from build123d import *

# Parameters (mm, degrees)
BOX024_W                = 6
BOX024_H                = 36
BOX024_DEPTH            = 23
CYLINDER011_R           = 2.75
CYLINDER011_DEPTH       = 74.5
CYLINDER011_PITCH_ANGLE = 90
CYLINDER008_R           = 1.75
CYLINDER008_DEPTH       = 21.5
CYLINDER008_PITCH_ANGLE = 90
CYLINDER009_R           = 3
CYLINDER009_DEPTH       = 21.5
CYLINDER009_PITCH_ANGLE = 90
BOX007_W                = 3
BOX007_H                = 56
BOX007_DEPTH            = 6
BOX008_W                = 3
BOX008_H                = 56
BOX008_DEPTH            = 6
BOX006_W                = 4
BOX006_H                = 56
BOX006_DEPTH            = 21
CYLINDER003_R           = 1.75
CYLINDER003_DEPTH       = 74.5
CYLINDER003_PITCH_ANGLE = 90
BOX003_W                = 28
BOX003_H                = 88
BOX003_DEPTH            = 38
BOX002_W                = 28
BOX002_H                = 88
BOX002_DEPTH            = 38
BOX001_W                = 47
BOX001_H                = 42
BOX001_DEPTH            = 25
BOX_W                   = 72
BOX_H                   = 58
BOX_DEPTH               = 24
FILLET_R                = 10
CHAMFER_SIZE            = 3


with BuildPart() as cube024:
    # Box024 → Box024 (new body)
    with BuildSketch(Plane(origin=(0, 19, 7), x_dir=(1, 0, 0), z_dir=(0, 0, 1))):
        with Locations((3, 18)):
            Rectangle(BOX024_W, BOX024_H)
    extrude(amount=BOX024_DEPTH)


with BuildPart() as joint_d013:
    # Cylinder011 → Cylinder011 (new body)
    with BuildSketch(Plane.XY):
        Circle(CYLINDER011_R)
    extrude(amount=CYLINDER011_DEPTH)


with BuildPart() as joint_d013_1:
    # Cylinder011 pitch: moved
    add(joint_d013.part.rotate(Axis((0, 0, 0), (0, 1, 0)), CYLINDER011_PITCH_ANGLE))


with BuildPart() as joint_d013_2:
    # Cylinder011 placement: moved
    add(joint_d013_1.part.moved(Location((-3, 9.5, 12))))


with BuildPart() as joint_d010:
    # Cylinder008 → Cylinder008 (new body)
    with BuildSketch(Plane.XY):
        Circle(CYLINDER008_R)
    extrude(amount=CYLINDER008_DEPTH)


with BuildPart() as joint_d010_1:
    # Cylinder008 pitch: moved
    add(joint_d010.part.rotate(Axis((0, 0, 0), (0, 1, 0)), CYLINDER008_PITCH_ANGLE))


with BuildPart() as joint_d010_2:
    # Cylinder008 placement: moved
    add(joint_d010_1.part.moved(Location((16, -24.5, 7))))


with BuildPart() as joint_d011:
    # Cylinder009 → Cylinder009 (new body)
    with BuildSketch(Plane.XY):
        Circle(CYLINDER009_R)
    extrude(amount=CYLINDER009_DEPTH)


with BuildPart() as joint_d011_1:
    # Cylinder009 pitch: moved
    add(joint_d011.part.rotate(Axis((0, 0, 0), (0, 1, 0)), CYLINDER009_PITCH_ANGLE))


with BuildPart() as joint_d011_2:
    # Cylinder009 placement: moved
    add(joint_d011_1.part.moved(Location((32, -24.5, 7))))


with BuildPart() as fusion001:
    # Fusion001 base: copy of Joint-D011
    add(joint_d011_2.part)

    # Fusion001: union Joint-D010
    add(joint_d010_2.part)


with BuildPart() as fusion002:
    # Fusion002 base: copy of Joint-D011
    add(joint_d011_2.part)

    # Fusion002: union Joint-D010
    add(joint_d010_2.part)


with BuildPart() as fusion002_1:
    # Fusion002 placement: moved
    add(fusion002.part.moved(Location((0, 0, 10))))


with BuildPart() as fusion003:
    # Fusion003 base: copy of Joint-D011
    add(joint_d011_2.part)

    # Fusion003: union Joint-D010
    add(joint_d010_2.part)


with BuildPart() as fusion003_1:
    # Fusion003 placement: moved
    add(fusion003.part.moved(Location((0, 49, 0))))


with BuildPart() as fusion004:
    # Fusion004 base: copy of Joint-D011
    add(joint_d011_2.part)

    # Fusion004: union Joint-D010
    add(joint_d010_2.part)


with BuildPart() as fusion004_1:
    # Fusion004 placement: moved
    add(fusion004.part.moved(Location((0, 49, 10))))


with BuildPart() as cube007:
    # Box007 → Box007 (new body)
    with BuildSketch(Plane(origin=(18.5, -28, 4), x_dir=(1, 0, 0), z_dir=(0, 0, 1))):
        with Locations((1.5, 28)):
            Rectangle(BOX007_W, BOX007_H)
    extrude(amount=BOX007_DEPTH)


with BuildPart() as cube008:
    # Box008 → Box008 (new body)
    with BuildSketch(Plane(origin=(18.5, -28, 14), x_dir=(1, 0, 0), z_dir=(0, 0, 1))):
        with Locations((1.5, 28)):
            Rectangle(BOX008_W, BOX008_H)
    extrude(amount=BOX008_DEPTH)


with BuildPart() as cube006:
    # Box006 → Box006 (new body)
    with BuildSketch(Plane(origin=(25.5, -28, 2), x_dir=(1, 0, 0), z_dir=(0, 0, 1))):
        with Locations((2, 28)):
            Rectangle(BOX006_W, BOX006_H)
    extrude(amount=BOX006_DEPTH)


with BuildPart() as joint_d005:
    # Cylinder003 → Cylinder003 (new body)
    with BuildSketch(Plane.XY):
        Circle(CYLINDER003_R)
    extrude(amount=CYLINDER003_DEPTH)


with BuildPart() as joint_d005_1:
    # Cylinder003 pitch: moved
    add(joint_d005.part.rotate(Axis((0, 0, 0), (0, 1, 0)), CYLINDER003_PITCH_ANGLE))


with BuildPart() as joint_d005_2:
    # Cylinder003 placement: moved
    add(joint_d005_1.part.moved(Location((-22, 9.5, 12))))


with BuildPart() as cube003:
    # Box003 → Box003 (new body)
    with BuildSketch(Plane(origin=(-33, -45, 1), x_dir=(1, 0, 0), z_dir=(0, 0, 1))):
        with Locations((14, 44)):
            Rectangle(BOX003_W, BOX003_H)
    extrude(amount=BOX003_DEPTH)


with BuildPart() as cube002:
    # Box002 → Box002 (new body)
    with BuildSketch(Plane(origin=(37, -45, 1), x_dir=(1, 0, 0), z_dir=(0, 0, 1))):
        with Locations((14, 44)):
            Rectangle(BOX002_W, BOX002_H)
    extrude(amount=BOX002_DEPTH)


with BuildPart() as cube001:
    # Box001 → Box001 (new body)
    with BuildSketch(Plane(origin=(-1, -21, 2), x_dir=(1, 0, 0), z_dir=(0, 0, 1))):
        with Locations((23.5, 21)):
            Rectangle(BOX001_W, BOX001_H)
    extrude(amount=BOX001_DEPTH)


with BuildPart() as pie_d:
    # Box → Box (new body)
    with BuildSketch(Plane(origin=(-15, -29, -3), x_dir=(1, 0, 0), z_dir=(0, 0, 1))):
        with Locations((36, 29)):
            Rectangle(BOX_W, BOX_H)
    extrude(amount=BOX_DEPTH)

    # Cut: cut Cube001
    add(cube001.part, mode=Mode.SUBTRACT)

    # Cut001: cut Cube002
    add(cube002.part, mode=Mode.SUBTRACT)

    # Cut002: cut Cube003
    add(cube003.part, mode=Mode.SUBTRACT)

    # Fillet
    fillet_edges = [pie_d.edges().sort_by_distance(p)[0] for p in [
        (-15, -29, -1),
        (-15, 29, -1),
        (57, -29, -1),
        (57, 29, -1),
    ]]
    fillet(fillet_edges, radius=FILLET_R)

    # Chamfer
    chamfer_edges = [pie_d.edges().sort_by_distance(p)[0] for p in [
        (-5, 0, 21),
        (37, 25, 21),
        (37, -25, 21),
    ]]
    chamfer(chamfer_edges, length=CHAMFER_SIZE)

    # Cut008: cut Joint-D005
    add(joint_d005_2.part, mode=Mode.SUBTRACT)

    # Cut010: cut Cube006
    add(cube006.part, mode=Mode.SUBTRACT)

    # Cut011: cut Cube008
    add(cube008.part, mode=Mode.SUBTRACT)

    # Cut012: cut Cube007
    add(cube007.part, mode=Mode.SUBTRACT)

    # Cut013: cut Fusion004
    add(fusion004_1.part, mode=Mode.SUBTRACT)

    # Cut014: cut Fusion003
    add(fusion003_1.part, mode=Mode.SUBTRACT)

    # Cut015: cut Fusion002
    add(fusion002_1.part, mode=Mode.SUBTRACT)

    # Cut016: cut Fusion001
    add(fusion001.part, mode=Mode.SUBTRACT)

    # Cut017: cut Joint-D013
    add(joint_d013_2.part, mode=Mode.SUBTRACT)

    # Cut039: cut Cube024
    add(cube024.part, mode=Mode.SUBTRACT)


with BuildPart() as pie_d_1:
    # Cut039 placement: moved
    add(pie_d.part.moved(Location((0, 0, 1))))


with BuildPart() as pie_i:
    # Part__Mirroring006: instance of pie-D
    add(pie_d_1.part.mirror(Plane(origin=(0, 0, 0), x_dir=(1, 0, 0), z_dir=(0, 1, 0))))


with BuildPart() as pie_i_1:
    # Part__Mirroring006 placement: moved
    add(pie_i.part.moved(Location((0, 72, 0))))


solid = pie_i_1.part
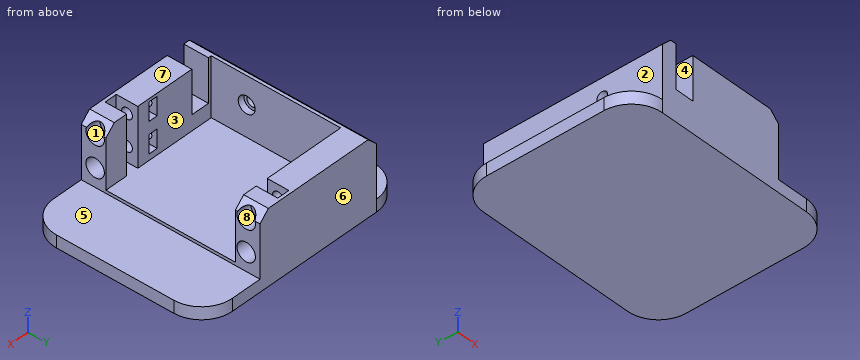
Here's how the part is built. I have some questions about the finished solid (model axes, mm). Face numbers are marked on the shaded views. A direction names the side the tool comes from. Round coordinates to 2 decimals unless told otherwise and drop trailing zeros. Write each loop counter-clockwise with the first axis right and the second up, starting at its lowest first coordinate (ties: lowest second). Pieces come first, ordered by that corner, then holes. Notation, with made-up numbers: (-21.5, 66) -> (31.5, 66) arc R7 cw to (31.5, 72) -> close; hole circle Ø6 at (-31, 80.25). An arc over 180 degrees is marked (long way). One line per item, written item: value.
1) Suppose I cut it at A-A on z = 13. List the corners of the cut face in (x, y) for me.
Filled sheet:
outline: (-5, 43) -> (0, 43) -> (0, 51) -> (-1, 51) -> (-1, 59.75) -> (-3, 59.75) -> (-3, 60.75) -> (-5, 60.75) -> close; (-5, 64.25) -> (-3, 64.25) -> (-3, 65.25) -> (-1, 65.25) -> (-1, 93) -> (25.5, 93) -> (25.5, 100) -> (29.5, 100) -> (29.5, 93) -> (37, 93) -> (37, 101) -> (-5, 101) -> close; (6, 43) -> (37, 43) -> (37, 51) -> (29.5, 51) -> (29.5, 44) -> (25.5, 44) -> (25.5, 51) -> (6, 51) -> close
2) Suppose I cut it at B-B on y = 62.5. List the corners of the cut face in (x, z) for me, plus the area to 4 significant figures.
Filled sheet:
outline: (-15, -2) -> (57, -2) -> (57, 2) -> (37, 2) -> (37, 3) -> (-1, 3) -> (-1, 10.25) -> (-3, 10.25) -> (-3, 11.25) -> (-5, 11.25) -> (-5, 2) -> (-15, 2) -> close; (-5, 14.75) -> (-3, 14.75) -> (-3, 15.75) -> (-1, 15.75) -> (-1, 22) -> (-2, 22) -> (-5, 19) -> close
area: 383.5 mm2
3) Suppose I cut it at C-C on y = 86. List the corners of the cut face in (x, z) for me.
Filled sheet:
outline: (-15, -2) -> (57, -2) -> (57, 2) -> (37, 2) -> (37, 3) -> (-1, 3) -> (-1, 22) -> (-2, 22) -> (-5, 19) -> (-5, 2) -> (-15, 2) -> close
4) If I drill on line 1 (Y direction, x = 17.1, z = 18); line 2 (Y direction, x = 34.2, z = 18); line 3 (Y direction, x = 29, z = 6.25), over which ranges is the centre line in solid material (lowest first)? Write a range as [from, to].
Filled sheet:
line 1: y = [43, 45.75], [49.25, 51], [93, 94.75], [98.25, 101]
line 2: y = [43, 44.5], [50.5, 51], [93, 93.5], [99.5, 101]
line 3: y = [43, 44], [100, 101]
5) Suppose I cut it at D-D on z = 4. List the corners of the cut face in (x, y) for me, plus the area to 3 significant figures.
Filled sheet:
outline: (-5, 43) -> (37, 43) -> (37, 51) -> (29.5, 51) -> (29.5, 44) -> (25.5, 44) -> (25.5, 51) -> (-1, 51) -> (-1, 93) -> (25.5, 93) -> (25.5, 100) -> (29.5, 100) -> (29.5, 93) -> (37, 93) -> (37, 101) -> (-5, 101) -> close
area: 784 mm2
6) For the marked faces 1, 2, 3, 4 and 5, which set-ups out of +Z, -Z, +X, -X, +Y, -Y let a thin tool reach every point of the face, with its end or its side?
Filled sheet:
face 1: +X
face 2: +Z, -X, +Y, -Y
face 3: +Z, +X
face 4: +Z, -Y
face 5: +Z, +X, +Y, -Y
7) I'm going to push flat-ended pins straight in: pin 1 Ø8 at (x, y) = (17, 67) entering from +Z; pin 2 Ø9 at (y, z) = (62.5, 13) entering from +X; pin 3 Ø12 at (y, z) = (86, 9) entering from -X. Where does each tip first touch, or does it pass through?
Filled sheet:
pin 1: stops at z = 3
pin 2: stops at x = -1
pin 3: stops at x = -5
8) We'd pull the mould along Y, two halves only. Please class the marked faces 6, 7 and 8: released by +Y, released by -Y, zero draft, split by the parting line, or undercut.
Filled sheet:
face 6: released by +Y
face 7: zero draft
face 8: undercut
